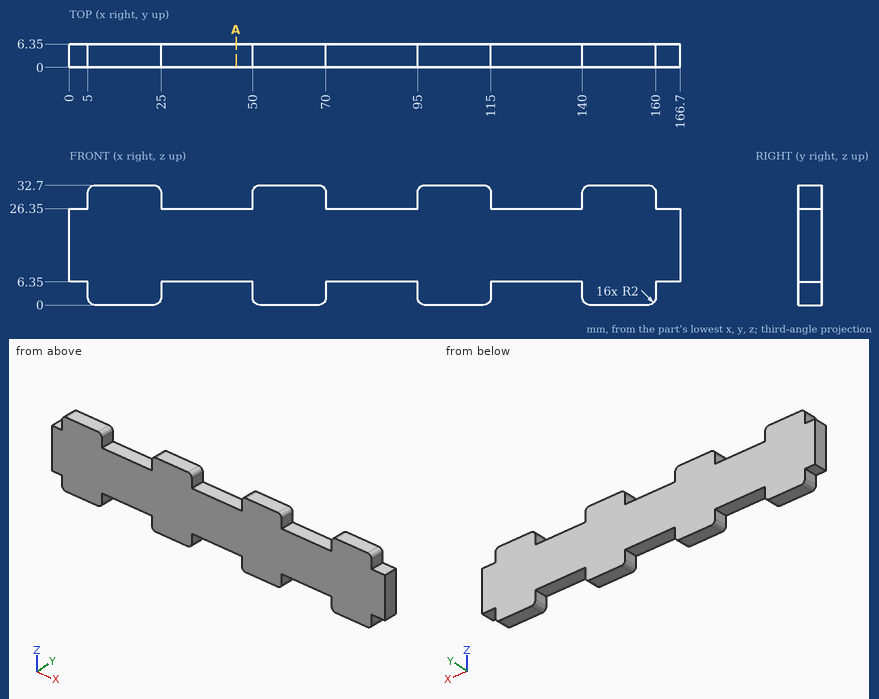
Source: three-view drawing plus pictorial views. Frame: mm from the lowest corner of the part. Round coordinates to 2 decimals unless told otherwise and drop trailing zeros. Loops run counter-clockwise (first coordinate to the right, second up) from the corner with the lowest first, then second, coordinate; pieces in that order, holes last.
Item 1: Line query: L1, parallel to X at y = 1.25, z = 4.5; L2, parallel to Z at x = 116.5, y = 3.25. Output: solid intervals per line, ascending.
Checked values:
L1: x = 5 to 25, 50 to 70, 95 to 115, 140 to 160
L2: z = 6.35 to 26.35
Item 2: Contact query for flat-ended pins moving along their axis: P1, Ø1, axis at y = 4, z = 4.5, coming from the -X side; P2, Ø1.9, axis at x = 79.5, y = 2.5, coming from the +Z side; P3, Ø1.3, axis at y = 2.5, z = 4.5, coming from the +X side. Output: stop coordinate, or through.
Checked values:
P1: stops at x = 5
P2: stops at z = 26.35
P3: stops at x = 160
Item 3: Section A-A, the plane x = 45.5. Output: boundary loops of the cut face in (y, z), plus the area to 3 significant figures.
Checked values:
outline: (0, 6.35) - (6.35, 6.35) - (6.35, 26.35) - (0, 26.35) - close
area: 127 mm2
